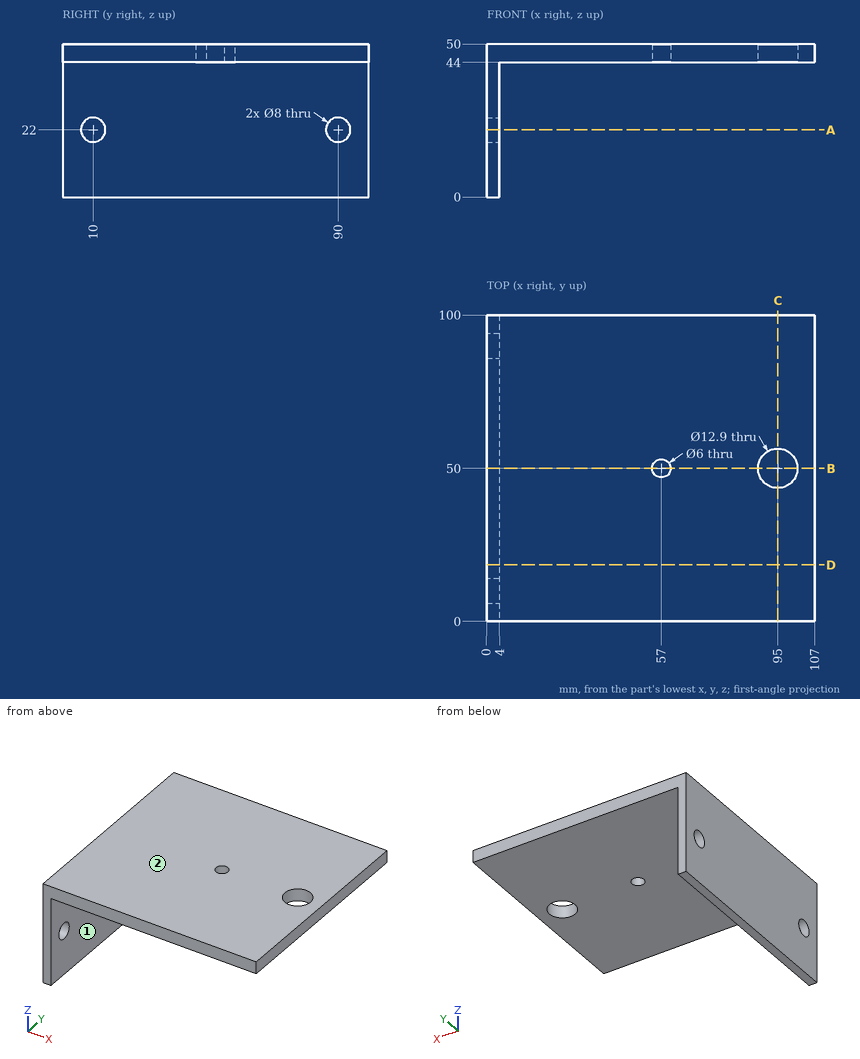
Input: dimensioned drawing with shaded views. Units: mm. Origin: part minimum x, y, z. A direction names the side the tool comes from. Give positions to 0.01 mm unless a question says otherwise; leave off trailing zeros. Loops run counter-clockwise (first coordinate to the right, second up) from the corner with the lowest first, then second, coordinate; pieces in that order, holes last. Notation, with made-up numbers: (-14.5, 83.5) -> (34.5, 83.5) arc R23 cw to (34.5, 119.5) -> close; hole circle Ø6 at (34, 79). An arc over 180 degrees is marked (long way). Return JSON: item names as keys, results as strings.
Item 1: Pin query (flat end, axial travel): P1, Ø10, axis at y = 46, z = 35.5, coming from the +X side; P2, Ø7, axis at y = 10, z = 22, coming from the -X side. Return the tip coordinate at first contact, or that it passes through.
Filled in:
{"P1": "x = 4", "P2": "through"}
Item 2: Section C-C, the plane x = 95. Output: boundary loops of the cut face in (y, z), plus the area to 3 significant figures.
Filled in:
{"outline": "(0, 44) -> (43.55, 44) -> (43.55, 50) -> (0, 50) -> close; (56.45, 44) -> (100, 44) -> (100, 50) -> (56.45, 50) -> close", "area": "523 mm^2"}
Item 3: Line query: line 1 (X direction, y = 50, z = 46.1); line 2 (Z direction, x = 2.65, y = 90); line 3 (X direction, y = 73.5, z = 19). Output: solid intervals per line, ascending.
Filled in:
{"line 1": "0 to 54, 60 to 88.55, 101.45 to 107", "line 2": "0 to 18, 26 to 50", "line 3": "0 to 4"}
Item 4: Section B-B, the plane y = 50. Output: boundary loops of the cut face in (x, z), plus the area to 3 significant figures.
Filled in:
{"outline": "(0, 0) -> (4, 0) -> (4, 44) -> (54, 44) -> (54, 50) -> (0, 50) -> close; (60, 44) -> (88.55, 44) -> (88.55, 50) -> (60, 50) -> close; (101.45, 44) -> (107, 44) -> (107, 50) -> (101.45, 50) -> close", "area": "705 mm^2"}
Item 5: Section D-D, the plane y = 18.5. Output: boundary loops of the cut face in (x, z), plus the area to 3 significant figures.
Filled in:
{"outline": "(0, 0) -> (4, 0) -> (4, 44) -> (107, 44) -> (107, 50) -> (0, 50) -> close", "area": "818 mm^2"}
Item 6: Section A-A, the plane z = 22. Output: boundary loops of the cut face in (x, y), plus the area to 3 significant figures.
Filled in:
{"outline": "(0, 0) -> (4, 0) -> (4, 6) -> (0, 6) -> close; (0, 14) -> (4, 14) -> (4, 86) -> (0, 86) -> close; (0, 94) -> (4, 94) -> (4, 100) -> (0, 100) -> close", "area": "336 mm^2"}
Item 7: Access query for the marked faces 1 and 2. Directions: +Z, -Z, +X, -X, +Y, -Y. A direction counts if a zero-diameter tool reaches every point of the face in a straight line with its end or side. Return the directions, or none.
Filled in:
{"face 1": "-Z, +X, +Y, -Y", "face 2": "+Z, +X, -X, +Y, -Y"}
